Source: CAD feature listing. Evaluate the final solid. Frame: model axes, mm. Coordinates: 2 decimals unless noted, no trailing zeros. Loops run counter-clockwise (first coordinate to the right, second up) from the corner with the lowest first, then second, coordinate; pieces in that order, holes last.
Item 1: Section query A-A, the plane x = 69. Return the cut outline in (y, z), then the cut area to 3 significant figures.
Item 2: Section query B-B, the plane x = 100. Return the cut outline in (y, z).
Item 3: Line query: probe 1 along Z at (x, y) = (264, 205); probe 2 along X at (y, z) = (110, 18.75). Output: solid intervals per line, ascending.
Item 4: Pin query (flat end, axial travel): pin 1 Ø5 at (x, z) = (178.5, 15.5) entering from +Y; pin 2 Ø8 at (x, y) = (112.5, 158.5) entering from +Z; pin 3 Ø3 at (x, z) = (127.5, 15) entering from -Y; pin 4 Ø8 at (x, z) = (134, 11.5) entering from -Y. Return the tip coordinate at first contact, or that it passes through.
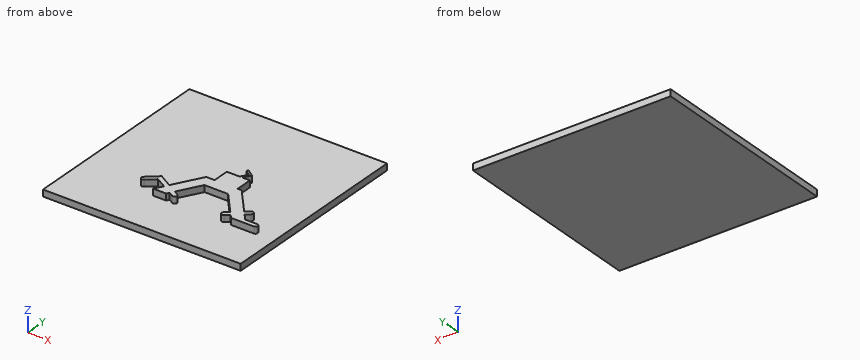
```python
from build123d import *

# Parameters (mm, degrees)
SKICA1_W                = 300
SKICA1_H                = 300
P_IDAT_VYSUNUT_M1_DEPTH = 10
P_IDAT_VYSUNUT_M3_DEPTH = 10


with BuildPart() as part:
    # Skica1 → Přidat vysunutím1 (new body)
    with BuildSketch(Plane.XY):
        with Locations((150, 150)):
            Rectangle(SKICA1_W, SKICA1_H)
    extrude(amount=P_IDAT_VYSUNUT_M1_DEPTH)

    # Skica3 → Přidat vysunutím3 (add)
    with BuildSketch(Plane.XY.offset(10)):
        with BuildLine():
            Line((116.91189832, 68), (124.126552838, 80.496148184))
            Line((124.126552838, 80.496148184), (108.180545378, 89.702579884))
            Line((108.180545378, 89.702579884), (95.03783106, 78.576572328))
            ThreePointArc((95.03783106, 78.576572328), (90.105085693, 78.986478585), (90.514991949, 83.919223952))
            Line((90.514991949, 83.919223952), (107.416046941, 98.226867031))
            Line((107.416046941, 98.226867031), (127.626552838, 86.55832601))
            Line((127.626552838, 86.55832601), (152.185045424, 129.094882926))
            Line((152.185045424, 129.094882926), (164.927230189, 129.094882926))
            Line((164.927230189, 129.094882926), (164.927230189, 154.094882926))
            Line((164.927230189, 154.094882926), (184.264906422, 154.094882926))
            Line((184.264906422, 154.094882926), (191.266981804, 164.094882926))
            Line((191.266981804, 164.094882926), (183.724437937, 169.376228999))
            ThreePointArc((183.724437937, 169.376228999), (183.356074525, 171.46532172), (185.445167246, 171.833685132))
            Line((185.445167246, 171.833685132), (195.445167246, 164.83160975))
            Line((195.445167246, 164.83160975), (187.927230189, 154.094882926))
            Line((187.927230189, 154.094882926), (199.927230189, 154.094882926))
            Line((199.927230189, 154.094882926), (199.927230189, 129.094882926))
            Line((199.927230189, 129.094882926), (205.927230189, 129.094882926))
            Line((205.927230189, 129.094882926), (238.917942598, 89.77808289))
            Line((238.917942598, 89.77808289), (245.046298143, 94.920383768))
            ThreePointArc((245.046298143, 94.920383768), (249.977210328, 94.488984851), (249.54581141, 89.558072666))
            Line((249.54581141, 89.558072666), (243.417455866, 84.415771788))
            Line((243.417455866, 84.415771788), (251.3182265, 75))
            Line((251.3182265, 75), (269.579798581, 75))
            ThreePointArc((269.579798581, 75), (273.079798581, 71.5), (269.579798581, 68))
            Line((269.579798581, 68), (235, 68))
            Line((235, 68), (230.394700333, 73.488382424))
            Line((230.394700333, 73.488382424), (224.266344788, 68.346081546))
            ThreePointArc((224.266344788, 68.346081546), (219.335432603, 68.777480463), (219.76683152, 73.708392648))
            Line((219.76683152, 73.708392648), (225.895187065, 78.850693526))
            Line((225.895187065, 78.850693526), (198, 112.094882926))
            Line((198, 112.094882926), (162, 112.094882926))
            Line((162, 112.094882926), (142.348984702, 78.05832601))
            Line((142.348984702, 78.05832601), (149.277187933, 74.05832601))
            ThreePointArc((149.277187933, 74.05832601), (150.558276846, 69.277237097), (145.777187933, 67.996148184))
            Line((145.777187933, 67.996148184), (138.848984702, 71.996148184))
            Line((138.848984702, 71.996148184), (136.541807473, 68))
            Line((136.541807473, 68), (116.91189832, 68))
        make_face()
    extrude(amount=P_IDAT_VYSUNUT_M3_DEPTH)


solid = part.part
```
Verdict:
1. outline: (0, 0) - (300, 0) - (300, 10) - (0, 10) - close
1. area: 3,000 mm2
2. outline: (0, 0) - (300, 0) - (300, 10) - (91.95, 10) - (91.95, 20) - (82.78, 20) - (82.78, 10) - (0, 10) - close
3. probe 1: z = 0 to 10
3. probe 2: x = 141.16 to 160.79, 199.76 to 221.95
4. pin 1: stops at y = 154.09
4. pin 2: stops at z = 10
4. pin 3: stops at y = 68
4. pin 4: stops at y = 0
